```python
from build123d import *

# Parameters (mm, degrees)
EXTRUDE_1_OUTLINE_W   = 88.8
EXTRUDE_1_OUTLINE_H   = 7.6
EXTRUDE_1_OUTLINE_W_2 = 7.6
EXTRUDE_1_OUTLINE_H_2 = 88.8
EXTRUDE_1_DEPTH       = 1
SKETCH_2_W            = 9.2
SKETCH_2_H            = 9.2
SKETCH_2_W_2          = 7.6
SKETCH_2_H_2          = 7.6
EXTRUDE_2_DEPTH       = 99


# Read off the part's stored shape, not the designer's step: 拉伸-薄壁1
with BuildPart() as part:
    # 拉伸-薄壁1 outline → 拉伸-薄壁1 (new body)
    with BuildSketch(Plane.XY):
        Polygon((-73.979591837, 5.816326531), (-73.979591837, -4.183673469), (26.020408163, -4.183673469), (26.020408163, 95.816326531), (16.020408163, 95.816326531), (16.020408163, 5.816326531), align=None)
        with Locations((-28.379591837, 0.816326531)):
            Rectangle(EXTRUDE_1_OUTLINE_W, EXTRUDE_1_OUTLINE_H, mode=Mode.SUBTRACT)
        with Locations((21.020408163, 0.816326531)):
            Rectangle(EXTRUDE_1_OUTLINE_W_2, EXTRUDE_1_OUTLINE_H, mode=Mode.SUBTRACT)
        with Locations((21.020408163, 50.216326531)):
            Rectangle(EXTRUDE_1_OUTLINE_W_2, EXTRUDE_1_OUTLINE_H_2, mode=Mode.SUBTRACT)
    extrude(amount=EXTRUDE_1_DEPTH)

    # 草图2 → 拉伸-薄壁2 (add)
    with BuildSketch(Plane.XY.offset(1)):
        with Locations((21.020408163, 0.816326531)):
            Rectangle(SKETCH_2_W, SKETCH_2_H)
        with Locations((21.020408163, 0.816326531)):
            Rectangle(SKETCH_2_W_2, SKETCH_2_H_2, mode=Mode.SUBTRACT)
    extrude(amount=EXTRUDE_2_DEPTH)


solid = part.part
```
Work out the finished part from the listing and answer in its coordinate system (mm). A direction names the side the tool comes from. Give positions to 0.01 mm unless a question says otherwise; leave off trailing zeros. Order: outer loops, then holes, each group sorted by start corner. A loop starts at its lowest first (then second) coordinate and runs counter-clockwise, first axis right, second up. Notation, with made-up numbers: (-16.75, -10.5) - (41.25, -10.5) arc R10 ccw to (41.25, -2.5) - close; hole circle Ø4 at (9.5, 12.5). An arc over 180 degrees is marked (long way). One line per item, written item: value. Start each with the question number.
1. Section C-C, the plane x = -38 is taken. Write down the section's boundary in (y, z).
2. Which of the six approach directions +Z, -Z, +X, -X, +Y, -Y give full straight-line access (tool end or side, diameter ignored) to faces 1 (the face through (25.62, 1, 50)), 2 (the face through (17.22, 1, 49)), 3 (the face through (16.42, 1, 50)), 4 (the face through (21, -3.784, 50)), 5 (the face through (-6, 5, 0))?
3. For a pull along Y with two mould halves and no side action, classify faces 6 (the face through (21, 5.416, 50)), 7 (the face through (25, 1, 100)), 8 (the face through (24.82, 1, 49)) as released by +Y, released by -Y, zero draft, split by the parting line, or undercut.
4. Section A-A, the plane z = 54.5 is taken. Write down the section's boundary in (x, y).
5. Section B-B, the plane y = 22 is taken. Write down the section's boundary in (x, z).
6. Each of these flat-tipped pins is pushed along its axis until it touches: pin 1 Ø0.8 at (y, z) = (47, 0.5) entering from -X; pin 2 Ø4 at (x, z) = (22, 34) entering from -Y; pin 3 Ø6 at (y, z) = (0, 56) entering from -X. Where does it stop, or does it pass through?
7. Consider line 1 (Y direction, x = 18.5, z = 95); line 2 (X direction, y = 3, z = 37); line 3 (Y direction, x = 17, z = 64.5). Determine where each line is inside the solid, lowest interval first.
Filled sheet:
1. outline: (-4.18, 0) - (-2.98, 0) - (-2.98, 1) - (-4.18, 1) - close; (4.62, 0) - (5.82, 0) - (5.82, 1) - (4.62, 1) - close
2. face 1: +Z, +X, +Y, -Y
2. face 2: +Z, -Z
2. face 3: +Z, -X, +Y, -Y
2. face 4: +Z, +X, -X, -Y
2. face 5: -Z, +X, -X, +Y, -Y
3. face 6: released by +Y
3. face 7: zero draft
3. face 8: undercut
4. outline: (16.42, -3.78) - (25.62, -3.78) - (25.62, 5.42) - (16.42, 5.42) - close; hole (17.22, -2.98) - (24.82, -2.98) - (24.82, 4.62) - (17.22, 4.62) - close
5. outline: (16.02, 0) - (17.22, 0) - (17.22, 1) - (16.02, 1) - close; (24.82, 0) - (26.02, 0) - (26.02, 1) - (24.82, 1) - close
6. pin 1: x = 16.02
6. pin 2: y = -3.78
6. pin 3: x = 16.42
7. line 1: -3.78 to -2.98, 4.62 to 5.42
7. line 2: 16.42 to 17.22, 24.82 to 25.62
7. line 3: -3.78 to 5.42
